Source: CAD feature listing. Evaluate the final solid. Frame: model axes, mm. A direction names the side the tool comes from. Coordinates: 2 decimals unless noted, no trailing zeros. Order: outer loops, then holes, each group sorted by start corner. A loop starts at its lowest first (then second) coordinate and runs counter-clockwise, first axis right, second up.
```python
from build123d import *

# Parameters (mm, degrees)
BOSS_EXTRUDE1_DEPTH = 8.552959
SKETCH2_W           = 8.552959
SKETCH2_H           = 14.1536931
BOSS_EXTRUDE2_DEPTH = 4


with BuildPart() as part:
    # Sketch1 → Boss-Extrude1 (new body)
    with BuildSketch(Plane.XY):
        Polygon((0, 0), (0, 14.1536931), (19.704590583, 14.1536931), (19.704590583, 8.1536931), (11.704590583, 8.1536931), (11.704590583, 6), (19.704590583, 6), (19.704590583, 0), align=None)
    extrude(amount=BOSS_EXTRUDE1_DEPTH)

    # Sketch2 → Boss-Extrude2 (add)
    with BuildSketch(Plane.ZY):
        with Locations((4.2764795, 7.07684655)):
            Rectangle(SKETCH2_W, SKETCH2_H)
    extrude(amount=BOSS_EXTRUDE2_DEPTH)


solid = part.part
```
Q1. Section query A-A on x = 16.75. Output: boundary loops of the cut face in (y, z), plus the area to 3 significant figures.
Solutions:
outline: (0, 0) - (6, 0) - (6, 8.55) - (0, 8.55) - close; (8.15, 0) - (14.15, 0) - (14.15, 8.55) - (8.15, 8.55) - close
area: 103 mm2
Q2. Section query B-B on z = 2.75. Output: boundary loops of the cut face in (x, y), plus the area to 3 significant figures.
Solutions:
outline: (-4, 0) - (19.7, 0) - (19.7, 6) - (11.7, 6) - (11.7, 8.15) - (19.7, 8.15) - (19.7, 14.15) - (-4, 14.15) - close
area: 318 mm2
Q3. Pull-direction query (Y, two-part tool) for faces 1 (the flat face through (-4, 7, 4)), 2 (the flat face through (16, 8.154, 4)), 3 (the flat face through (8, 14.154, 4)); classes: pulls with the +Y half, pulls with the -Y half, needs draft (parallel to the pull), parting line crosses it, or undercut.
Solutions:
face 1: needs draft
face 2: undercut
face 3: pulls with the +Y half
Q4. Pin query (flat end, axial travel): P1, Ø1.1, axis at y = 7, z = 5, coming from the +X side. Return the tip coordinate at first contact, or that it passes through.
Solutions:
P1: stops at x = 11.7
Q5. Set-up query: faces 4 (the flat face through (11.705, 7, 4)), 5 (the flat face through (19.705, 3, 4)). Return all of +Z, -Z, +X, -X, +Y, -Y with unobstructed straight access to the full face (end or side cutting, diameter ignored); none if empty.
Solutions:
face 4: +Z, -Z, +X
face 5: +Z, -Z, +X, +Y, -Y
Q6. Material intervals for line 1 along Y through (x, z) = (12.25, 6.5); line 2 along X through (y, z) = (7.25, 0.5), sorted ascending.
Solutions:
line 1: y = 0 to 6, 8.15 to 14.15
line 2: x = -4 to 11.7
